Input: part model. Units: mm. Frame: model coordinates. Face numbers are marked on the shaded views. A direction names the side the tool comes from. Give positions to 0.01 mm unless a question says otherwise; leave off trailing zeros. Loops run counter-clockwise (first coordinate to the right, second up) from the corner with the lowest first, then second, coordinate; pieces in that order, holes last. Notation, with made-up numbers: (35, -3) - (40, -3) arc R36 ccw to (40, 33) - close; hole circle Ø11 at (-12.5, 13). An arc over 180 degrees is marked (long way). One line per question, with ' | ' between items. Start each with the question number.
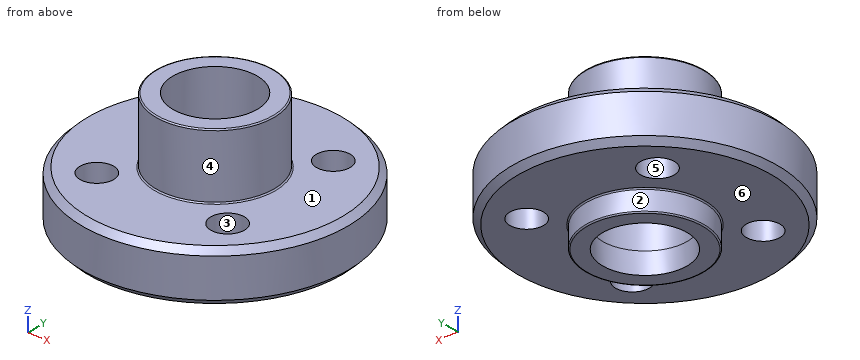
from build123d import *

# Parameters (mm, degrees)
F0_R          = 11
F0_R_2        = 1.4
F0_R_3        = 4.9
F0_R_4        = 3.5
F1_DEPTH      = 4.22
F2_DEPTH      = 5.4
F2_DEPTH_BACK = 6
F3_SIZE       = 0.5
F4_R          = 0.1


with BuildPart() as f1:
    # F0 (on Top) → F1 (new body)
    with BuildSketch(Plane.XY):
        Circle(F0_R)
        with Locations((-5.374011537, -5.374011537)):
            Circle(F0_R_2, mode=Mode.SUBTRACT)
        with Locations((5.374011537, -5.374011537)):
            Circle(F0_R_2, mode=Mode.SUBTRACT)
        with Locations((-5.374011537, 5.374011537)):
            Circle(F0_R_2, mode=Mode.SUBTRACT)
        Circle(F0_R_3, mode=Mode.SUBTRACT)
        with Locations((5.374011537, 5.374011537)):
            Circle(F0_R_2, mode=Mode.SUBTRACT)
        Circle(F0_R_3)
        Circle(F0_R_4, mode=Mode.SUBTRACT)
    extrude(amount=-F1_DEPTH)

    # F0 (on Top) → F2 (join, two sides)
    with BuildSketch(Plane.XY) as f2_sk:
        Circle(F0_R_3)
        Circle(F0_R_4, mode=Mode.SUBTRACT)
    extrude(amount=F2_DEPTH)
    extrude(f2_sk.sketch, amount=-F2_DEPTH_BACK)

    # F3
    f3_edges = [f1.edges().sort_by_distance(p)[0] for p in [
        (-11, 0, 0),
        (-11, 0, -4.22),
    ]]
    chamfer(f3_edges, length=F3_SIZE)

    # F4
    f4_edges = [f1.edges().sort_by_distance(p)[0] for p in [
        (-4.9, 0, 5.4),
        (-4.9, 0, 0),
        (-4.9, 0, -4.22),
        (-4.9, 0, -6),
    ]]
    fillet(f4_edges, radius=F4_R)


solid = f1.part
Q1. Section D-D, the plane z = 0.75. Output: boundary loops of the cut face in (x, y), plus the area to 3 significant figures.
Q2. Section C-C, the plane z = -2.5. Output: boundary loops of the cut face in (x, y).
Q3. Access query for the marked faces 4, 5 and 6. Directions: +Z, -Z, +X, -X, +Y, -Y. A direction counts if a zero-diameter tool reaches every point of the face in a straight line with its end or side. Return the directions, or none.
Q4. Section A-A, the plane y = 0. Output: boundary loops of the cut face in (x, z), plus the area to 3 significant figures.
Q5. Line query: L1, parallel to Y at x = 0, z = -5.55; L2, parallel to Y at x = 0, z = -1.5; L3, parallel to Y at x = -5.5, z = -2.25. Output: solid intervals per line, ascending. Write a range as from..to.
Q6. First-contact query: pin 1 (2 mm diameter, centred on x = 5.37, y = -5.37, fed in from -Z); pin 2 (4 mm diameter, centred on x = -3.5, z = 0.5, fed in from +Y); pin 3 (5 mm diameter, centred on x = -7, y = 3.5, fed in from +Z); pin 4 (8 mm diameter, centred on x = 6, y = 6, fed in from -Z). Flat tips, straight axial feed; report the tip coordinate or a pass-through.
Q7. Draft query along Y for the marked faces 1, 2 and 3. Return one class per face: +Y half, -Y half, draft (parallel to the pull), parting line (faces both ways), or undercut.
Solved:
1) outline: circle Ø9.8 at (0, 0); hole circle Ø7 at (0, 0) | area: 36.9 mm²
2) outline: circle Ø22 at (0, 0); hole circle Ø2.8 at (-5.37, -5.37); hole circle Ø2.8 at (-5.37, 5.37); hole circle Ø7 at (0, 0); hole circle Ø2.8 at (5.37, -5.37); hole circle Ø2.8 at (5.37, 5.37)
3) face 4: +Z | face 5: +Z, -Z | face 6: -Z
4) outline: (-11, -3.72) - (-10.5, -4.22) - (-5, -4.22) arc R0.1 cw to (-4.9, -4.32) - (-4.9, -5.9) arc R0.1 ccw to (-4.8, -6) - (-3.5, -6) - (-3.5, 5.4) - (-4.8, 5.4) arc R0.1 ccw to (-4.9, 5.3) - (-4.9, 0.1) arc R0.1 cw to (-5, 0) - (-10.5, 0) - (-11, -0.5) - close; (3.5, -6) - (4.8, -6) arc R0.1 ccw to (4.9, -5.9) - (4.9, -4.32) arc R0.1 cw to (5, -4.22) - (10.5, -4.22) - (11, -3.72) - (11, -0.5) - (10.5, 0) - (5, 0) arc R0.1 cw to (4.9, 0.1) - (4.9, 5.3) arc R0.1 ccw to (4.8, 5.4) - (3.5, 5.4) - close | area: 82.9 mm²
5) L1: y = -4.9..-3.5, 3.5..4.9 | L2: y = -11..-3.5, 3.5..11 | L3: y = -9.53..-6.77, -3.98..3.98, 6.77..9.53
6) pin 1: passes through | pin 2: stops at y = 10.86 | pin 3: stops at z = 0 | pin 4: stops at z = -6
7) face 1: draft | face 2: parting line | face 3: undercut
